from build123d import *

# Parameters (mm, degrees)
SKETCH1_W            = 89
SKETCH1_H            = 192
BOSS_EXTRUDE1_DEPTH  = 30
SKETCH2_R            = 34.99943994
CUT_EXTRUDE1_DEPTH   = 10
SKETCH3_W            = 75
SKETCH3_H            = 5
CUT_EXTRUDE2_DEPTH   = 102
CUT_EXTRUDE4_DEPTH   = 102
SKETCH6_W            = 10.5
SKETCH6_H            = 4
CUT_EXTRUDE7_DEPTH   = 8
BOSS_EXTRUDE2_DEPTH  = 10.5
CUT_EXTRUDE8_DEPTH   = 20.767757578
BOSS_EXTRUDE3_DEPTH  = 10.5
CUT_EXTRUDE9_DEPTH   = 22.812544275
BOSS_EXTRUDE6_DEPTH  = 10.5
BOSS_EXTRUDE7_DEPTH  = 10.5
FILLET1_R            = 10
FILLET2_R            = 10
FILLET3_R            = 10
FILLET4_R            = 10
CUT_EXTRUDE11_DEPTH  = 99
SKETCH15_W           = 7.554212703
SKETCH15_H           = 3.259234926
CUT_EXTRUDE12_DEPTH  = 99
FILLET5_R            = 10
SKETCH16_W           = 4.893814379
SKETCH16_H           = 8
BOSS_EXTRUDE8_DEPTH  = 4
SKETCH17_R           = 2
CUT_EXTRUDE13_DEPTH  = 4
SKETCH18_W           = 192
SKETCH18_H           = 3
BOSS_EXTRUDE9_DEPTH  = 5
SKETCH19_W           = 192
SKETCH19_H           = 3
BOSS_EXTRUDE10_DEPTH = 5


with BuildPart() as part:
    # Sketch1 → Boss-Extrude1 (new body)
    with BuildSketch(Plane(origin=(0, 0, 0), x_dir=(1, 0, 0), z_dir=(0, 1, 0))):
        with Locations((-10.5, 20.043668932)):
            Rectangle(SKETCH1_W, SKETCH1_H)
        with BuildLine():
            Line((-44.5, -34.956331068), (-44.5, 75.043668932))
            ThreePointArc((-44.5, 75.043668932), (-10.5, 109.043668932), (23.5, 75.043668932))
            Line((23.5, 75.043668932), (23.5, -34.956331068))
            ThreePointArc((23.5, -34.956331068), (-10.5, -68.956331068), (-44.5, -34.956331068))
        make_face(mode=Mode.SUBTRACT)
    extrude(amount=BOSS_EXTRUDE1_DEPTH)

    # Sketch2 → Cut-Extrude1 (cut)
    with BuildSketch(Plane.XZ):
        with Locations((-10.5, 37.838844027)):
            Circle(SKETCH2_R)
    extrude(amount=-CUT_EXTRUDE1_DEPTH, mode=Mode.SUBTRACT)

    # Sketch3 → Cut-Extrude2 (cut)
    with BuildSketch(Plane(origin=(34, 0, 0), x_dir=(0, 0, -1), z_dir=(1, 0, 0))):
        with Locations((-34.286288065, 12.5)):
            Rectangle(SKETCH3_W, SKETCH3_H)
    extrude(amount=-CUT_EXTRUDE2_DEPTH, mode=Mode.SUBTRACT)

    # Sketch4 → Cut-Extrude4 (cut)
    with BuildSketch(Plane.ZY.offset(55)):
        Polygon((-40.970715348, 29.469395922), (-41.211628541, 24.561719678), (-3.213711935, 10), (-3.213711935, 15), align=None)
    extrude(amount=-CUT_EXTRUDE4_DEPTH, mode=Mode.SUBTRACT)

    # Sketch6 → Cut-Extrude7 (cut)
    with BuildSketch(Plane(origin=(0, 30, 0), x_dir=(1, 0, 0), z_dir=(0, 1, 0))):
        with Locations((-49.75, 40.570603007)):
            Rectangle(SKETCH6_W, SKETCH6_H)
        with Locations((28.75, 40.570603007)):
            Rectangle(SKETCH6_W, SKETCH6_H)
    extrude(amount=-CUT_EXTRUDE7_DEPTH, mode=Mode.SUBTRACT)

    # Sketch7 → Boss-Extrude2 (add)
    with BuildSketch(Plane.ZY.offset(55)):
        Polygon((-38.570603007, 23.549614886), (-42.570603007, 25.082511526), (-42.570603007, 22), (-38.570603007, 22), align=None)
    extrude(amount=-BOSS_EXTRUDE2_DEPTH)

    # Sketch8 → Cut-Extrude8 (cut)
    with BuildSketch(Plane.ZY.offset(55)):
        Polygon((-42.570603007, 25.082511526), (-55.402488324, 30), (-42.570603007, 30), align=None)
    extrude(amount=-CUT_EXTRUDE8_DEPTH, mode=Mode.SUBTRACT)

    # Sketch9 → Boss-Extrude3 (add)
    with BuildSketch(Plane(origin=(34, 0, 0), x_dir=(0, 0, -1), z_dir=(1, 0, 0))):
        Polygon((38.570603007, 23.549614886), (42.570603007, 25.082511526), (42.570603007, 22), (38.570603007, 22), align=None)
    extrude(amount=-BOSS_EXTRUDE3_DEPTH)

    # Sketch10 → Cut-Extrude9 (cut)
    with BuildSketch(Plane(origin=(34, 0, 0), x_dir=(0, 0, -1), z_dir=(1, 0, 0))):
        Polygon((42.570603007, 25.082511526), (55.402488324, 30), (42.570603007, 30), align=None)
    extrude(amount=-CUT_EXTRUDE9_DEPTH, mode=Mode.SUBTRACT)

    # Sketch12 → Boss-Extrude6 (add)
    with BuildSketch(Plane.ZY.offset(55)):
        Polygon((-38.570603007, 30), (-41.570603007, 30), (-38.570603007, 28.549614886), align=None)
    extrude(amount=-BOSS_EXTRUDE6_DEPTH)

    # Sketch11 → Boss-Extrude7 (add)
    with BuildSketch(Plane(origin=(34, 0, 0), x_dir=(0, 0, -1), z_dir=(1, 0, 0))):
        Polygon((38.570603007, 28.549614886), (41.570603007, 30.007074027), (38.570603007, 30), align=None)
    extrude(amount=-BOSS_EXTRUDE7_DEPTH)

    # Fillet1
    fillet1_edges = [part.edges().sort_by_distance(p)[0] for p in [
        (-49.75, 30, -55.402488324),
    ]]
    fillet(fillet1_edges, radius=FILLET1_R)

    # Fillet2
    fillet2_edges = [part.edges().sort_by_distance(p)[0] for p in [
        (28.75, 30, -55.402488324),
    ]]
    fillet(fillet2_edges, radius=FILLET2_R)

    # Fillet3
    fillet3_edges = [part.edges().sort_by_distance(p)[0] for p in [
        (-49.75, 10, -3.213711935),
    ]]
    fillet(fillet3_edges, radius=FILLET3_R)

    # Fillet4
    fillet4_edges = [part.edges().sort_by_distance(p)[0] for p in [
        (28.75, 10, -3.213711935),
    ]]
    fillet(fillet4_edges, radius=FILLET4_R)

    # Sketch14 → Cut-Extrude11 (cut)
    with BuildSketch(Plane(origin=(34, 0, 0), x_dir=(0, 0, -1), z_dir=(1, 0, 0))):
        Polygon((42.717415751, 25.138773717), (116.043668932, 25.138773717), (116.043668932, 30), (57.252994033, 30), (53.674522762, 29.337801849), align=None)
    extrude(amount=-CUT_EXTRUDE11_DEPTH, mode=Mode.SUBTRACT)


with BuildPart() as cut_extrude11_piece_1:
    # of the separate pieces the step leaves, piece 1, a body of its own (cut_extrude11_pieces)
    add(part.part.solids().sort_by_distance((23.5, 25.138773717, -42.717415751))[0])

    # Fillet5
    fillet5_edges = [cut_extrude11_piece_1.edges().sort_by_distance(p)[0] for p in [
        (-49.75, 25.138773717, -42.717415751),
        (28.75, 25.138773717, -42.717415751),
    ]]
    fillet(fillet5_edges, radius=FILLET5_R)

    # Sketch16 → Boss-Extrude8 (add)
    with BuildSketch(Plane(origin=(0, 0, 0), x_dir=(0, 0, -1), z_dir=(1, 0, 0))):
        with Locations((118.490576121, 11.138773717)):
            Rectangle(SKETCH16_W, SKETCH16_H)
    extrude(amount=BOSS_EXTRUDE8_DEPTH)

    # Sketch17 → Cut-Extrude13 (cut)
    with BuildSketch(Plane(origin=(4, 0, 0), x_dir=(0, 0, -1), z_dir=(1, 0, 0))):
        with Locations(Location((117.893374439, 11.138773717, 0), (0, 0, 202.353838102))):
            Circle(SKETCH17_R)
    extrude(amount=-CUT_EXTRUDE13_DEPTH, mode=Mode.SUBTRACT)

    # Sketch18 → Boss-Extrude9 (add)
    with BuildSketch(Plane(origin=(34, 0, 0), x_dir=(0, 0, -1), z_dir=(1, 0, 0))):
        with Locations((20.043668932, 1.5)):
            Rectangle(SKETCH18_W, SKETCH18_H)
    extrude(amount=BOSS_EXTRUDE9_DEPTH)

    # Sketch19 → Boss-Extrude10 (add)
    with BuildSketch(Plane.ZY.offset(55)):
        with Locations((-20.043668932, 1.5)):
            Rectangle(SKETCH19_W, SKETCH19_H)
    extrude(amount=BOSS_EXTRUDE10_DEPTH)


with BuildPart() as cut_extrude11_piece_2:
    # of the separate pieces the step leaves, piece 2, a body of its own (cut_extrude11_pieces)
    add(part.part.solids().sort_by_distance((23.5, 30, -57.252994033))[0])


with BuildPart() as cut_extrude11_piece_3:
    # of the separate pieces the step leaves, piece 3, a body of its own (cut_extrude11_pieces)
    add(part.part.solids().sort_by_distance((-55, 30, -57.252994033))[0])


with BuildPart() as cut_extrude12_tool:
    # Sketch15 → Cut-Extrude12 (new body)
    with BuildSketch(Plane(origin=(34, 0, 0), x_dir=(0, 0, -1), z_dir=(1, 0, 0))):
        with Locations((54.846987071, 29.864387296)):
            Rectangle(SKETCH15_W, SKETCH15_H)
    extrude(amount=-CUT_EXTRUDE12_DEPTH)


with BuildPart() as cut_extrude11_piece_2_1:
    add(cut_extrude11_piece_2.part)

    # Cut-Extrude12: cut by cut_extrude12_tool
    add(cut_extrude12_tool.part, mode=Mode.SUBTRACT)


with BuildPart() as cut_extrude11_piece_3_1:
    add(cut_extrude11_piece_3.part)

    # Cut-Extrude12: cut by cut_extrude12_tool
    add(cut_extrude12_tool.part, mode=Mode.SUBTRACT)


solid = cut_extrude11_piece_1.part
Could you check a few things on this model? Use its own coordinates, in mm. A direction names the side the tool comes from. Coordinates: 2 decimals unless noted, no trailing zeros. Write each loop counter-clockwise with the first axis right and the second up, starting at its lowest first coordinate (ties: lowest second). Pieces come first, ordered by that corner, then holes. Notation, with made-up numbers: (83.25, -9) - (113.25, -9) arc R25 cw to (113.25, 28) - close; hole circle Ø10 at (58, -18). An arc over 180 degrees is marked (long way). Write item = value, one per line.
1) Please list where these lines run through material, in increasing order: line 1 (X direction, y = 23.5, z = -72); line 2 (Z direction, x = -10, y = 5); line 3 (Z direction, x = -9, y = 25). Write a range as [from, to].
Result set:
line_1 = [-55, -44.5], [23.5, 34]
line_2 = [-116.04, -109.04], [72.83, 75.96]
line_3 = [-116.04, -109.01], [68.92, 75.96]
2) Suppose I cut it at C-C on z = -29. Please give me the cut outline in (x, y).
Result set:
outline = (-60, 0) - (-44.5, 0) - (-44.5, 19.88) - (-55, 19.88) - (-55, 3) - (-60, 3) - close; (-55, 24.88) - (-44.5, 24.88) - (-44.5, 30) - (-55, 30) - close; (23.5, 0) - (39, 0) - (39, 3) - (34, 3) - (34, 19.88) - (23.5, 19.88) - close; (23.5, 24.88) - (34, 24.88) - (34, 30) - (23.5, 30) - close
3) Will these pins go through, and if not, where does the flat tip stop? pin 1 Ø16.5 at (y, z) = (23, -10) entering from +X; pin 2 Ø3 at (y, z) = (24, -6) entering from -X; pin 3 Ø1 at (x, y) = (0, 17.5) entering from -Z; pin 4 Ø1.2 at (x, z) = (-12, 72.5) entering from -Y.
Result set:
pin_1 = 34
pin_2 = -55
pin_3 = -116.04
pin_4 = 0
4) We'd pull the mould along Z, two halves only. Please class faces 1 (the flat face through (-10, 12, 71.786)), 2 (the flat face through (2, 11, -120.937)), 3 (the flat face through (0, 11.2, -120.1)): +Z half, -Z half, draft (parallel to the pull), parting line (faces both ways), or undercut.
Result set:
face_1 = undercut
face_2 = -Z half
face_3 = draft
5) Suppose I cut it at A-A on x = -10.5. Please give me the cut outline in (y, z), plus the area to 3 significant figures.
Result set:
outline = (0, -116.04) - (25.14, -116.04) - (25.14, -109.04) - (0, -109.04) - close; (0, 72.84) - (10, 72.84) - (10, 71.79) - (15, 71.79) - (15, 68.96) - (30, 68.96) - (30, 75.96) - (0, 75.96) - close
area = 333 mm2
6) Suppose I cut it at B-B on z = -92.5. Please give me the cut outline in (x, y).
Result set:
outline = (-60, 0) - (-39.68, 0) - (-39.68, 25.14) - (-55, 25.14) - (-55, 3) - (-60, 3) - close; (18.68, 0) - (39, 0) - (39, 3) - (34, 3) - (34, 25.14) - (18.68, 25.14) - close
7) For faces 4 (the cylindrical face through (-9.613, 4.93, 72.827)), 5 (the flat face through (2, 7.139, -118)), 6 (the flat face through (-55, 16.7, -21.4)), 7 (the flat face through (-49, 10, 44)), 8 (the flat face through (-44.5, 23, 5)), which set-ups out of +Z, -Z, +X, -X, +Y, -Y let a thin tool reach every point of the face, with its end or its side?
Result set:
face_4 = -Y
face_5 = -Z, +X, -X, -Y
face_6 = +Z, -Z, -X, +Y
face_7 = +X, -X
face_8 = +Y, -Y
